Here's how the part is built. I have some questions about the finished solid (model axes, mm). A direction names the side the tool comes from. Round coordinates to 2 decimals unless told otherwise and drop trailing zeros. Order: outer loops, then holes, each group sorted by start corner. A loop starts at its lowest first (then second) coordinate and runs counter-clockwise, first axis right, second up. Notation, with made-up numbers: (67.25, 88) -> (104.25, 88) arc R22 cw to (104.25, 120) -> close; hole circle Ø2 at (-5, 74.5). An arc over 180 degrees is marked (long way). One line per item, written item: value.
```python
from build123d import *

# Parameters (mm, degrees)
SKETCH_1_W             = 7.62
SKETCH_1_H             = 7.3
EXTRUDE_1_DEPTH        = 8.6
CHAMFER_1_SIZE         = 2
SKETCH_2_W             = 1.5
SKETCH_2_H             = 2.244760595
CUT_EXTRUDE_1_DEPTH    = 0.5
PATTERN_LINEAR_1_COUNT = 2
PATTERN_LINEAR_1_PITCH = 3.81
SKETCH_3_R             = 0.6
EXTRUDE_2_DEPTH        = 3.4
PATTERN_LINEAR_2_COUNT = 2
PATTERN_LINEAR_2_PITCH = 3.81


with BuildPart() as part:
    # 草图1 → 凸台-拉伸1 (new body)
    with BuildSketch(Plane.XY):
        with Locations((3.81, 3.65)):
            Rectangle(SKETCH_1_W, SKETCH_1_H)
    extrude(amount=EXTRUDE_1_DEPTH)

    # 倒角1
    chamfer_1_edges = [part.edges().sort_by_distance(p)[0] for p in [
        (3.81, 7.3, 8.6),
        (3.81, 0, 8.6),
    ]]
    chamfer(chamfer_1_edges, length=CHAMFER_1_SIZE)

    # 草图2 → 切除-拉伸1 (cut)
    with BuildSketch(Plane.XZ):
        with Locations((1.905, 3.602057757)):
            Rectangle(SKETCH_2_W, SKETCH_2_H)
    cut_extrude_1 = extrude(amount=-CUT_EXTRUDE_1_DEPTH, mode=Mode.SUBTRACT)

    # 阵列(线性)1: 切除-拉伸1 ×2
    with Locations(*[(i * PATTERN_LINEAR_1_PITCH, 0, 0) for i in range(1, PATTERN_LINEAR_1_COUNT)]):
        add(cut_extrude_1, mode=Mode.SUBTRACT)

    # 草图3 → 凸台-拉伸2 (add)
    with BuildSketch(Plane(origin=(0, 0, 0), x_dir=(-1, 0, 0), z_dir=(0, 0, -1))):
        with Locations((-5.715, 3.7)):
            Circle(SKETCH_3_R)
    extrude_2 = extrude(amount=EXTRUDE_2_DEPTH)

    # 阵列(线性)2: 凸台-拉伸2 ×2
    with Locations(*[(-i * PATTERN_LINEAR_2_PITCH, 0, 0) for i in range(1, PATTERN_LINEAR_2_COUNT)]):
        add(extrude_2)


solid = part.part
```
Q1. If we mould it in two halves opening along X, with no side actions, what happens to faces 1 (the face through (4, 4, 8.6)), 2 (the face through (7.62, 4, 4)), 3 (the face through (2, 0.5, 4)), 4 (the face through (0, 4, 4))? For each: pulls with the +X half, pulls with the -X half, needs draft (parallel to the pull), parting line crosses it, or undercut.
Answers:
face 1: needs draft
face 2: pulls with the +X half
face 3: undercut
face 4: pulls with the -X half
Q2. Which directions (+Z, -Z, +X, -X, +Y, -Y) give clear straight access to the entire face, cutting with the end or side of a thin tool? Please do faces 5 (the face through (5.845, 3.114, -1.676)), 6 (the face through (6, 0.5, 4)), 7 (the face through (3.8, 6.3, 7.6)).
Answers:
face 5: -Z
face 6: -Y
face 7: +Z, +X, -X, +Y
Q3. I want a section at A-A on z = -1.5. Write out the boundary of the cut face in (x, y) (3 decimals).
Answers:
outline: circle Ø1.2 at (1.905, 3.7); circle Ø1.2 at (5.715, 3.7)
Q4. I want a section at B-B on y = 3.7. Write out the boundary of the cut face in (x, z) (3 decimals), then the cut area to 3 significant figures.
Answers:
outline: (0, 0) -> (1.305, 0) -> (1.305, -3.4) -> (2.505, -3.4) -> (2.505, 0) -> (5.115, 0) -> (5.115, -3.4) -> (6.315, -3.4) -> (6.315, 0) -> (7.62, 0) -> (7.62, 8.6) -> (0, 8.6) -> close
area: 73.7 mm2
Q5. I need wall thicknesses on line 1 along Z through (x, y) = (1.75, 2.25); line 2 along Y through (x, z) = (2.25, 3.75); line 3 along Y through (x, z) = (7, 6.75). Which ranges of each line are inside material? Lowest first, please.
Answers:
line 1: 0 to 8.6
line 2: 0.5 to 7.3
line 3: 0.15 to 7.15
Q6. I want a section at C-C on z = 3.25. Write out the boundary of the cut face in (x, y) (3 decimals), then the cut area to 3 significant figures.
Answers:
outline: (0, 0) -> (1.155, 0) -> (1.155, 0.5) -> (2.655, 0.5) -> (2.655, 0) -> (4.965, 0) -> (4.965, 0.5) -> (6.465, 0.5) -> (6.465, 0) -> (7.62, 0) -> (7.62, 7.3) -> (0, 7.3) -> close
area: 54.1 mm2
Q7. For P1, Ø1.5, axis at x = 4, y = 4.5, coming from the -Z side; P2, Ø0.5, axis at x = 2, z = 3.5, coming from the -Y side; P3, Ø0.6, axis at x = 2, y = 0.5, coming from the +Z side, each with a flat end and sliding along its axis, tell me the tip position at first contact or that it passes through.
Answers:
P1: z = 0
P2: y = 0.5
P3: z = 7.4
Q8. I want a section at D-D on x = 4. Write out the boundary of the cut face in (y, z).
Answers:
outline: (0, 0) -> (7.3, 0) -> (7.3, 6.6) -> (5.3, 8.6) -> (2, 8.6) -> (0, 6.6) -> close
